Verification items for the finished model (mm, model axes). Round coordinates to 2 decimals unless told otherwise and drop trailing zeros. Order: outer loops, then holes, each group sorted by start corner. A loop starts at its lowest first (then second) coordinate and runs counter-clockwise, first axis right, second up. Notation, with made-up numbers: (66.25, 5.5) -> (80.25, 5.5) arc R20 ccw to (80.25, 22.5) -> close; hole circle Ø7 at (74, 59). An arc over 180 degrees is marked (long way). Return JSON: item names as keys, results as strings. Group by question number.
1) Section check A-A on y = -4. Enter the section's corners in (x, z) (3 decimals), plus the area to 3 significant figures.
2) Depth check by flat-ended pin: pin 1 (1.5 mm diameter, centred on x = -0.5, y = -1.5, fed in from +Z). Enter the tip coordinate at first touch or a pass-through.
3) Scan lines: L1, parallel to Z at x = -0.05, y = -5.25; L2, parallel to Y at x = -0.85, z = 0.65; L3, parallel to Z at x = -0.8, y = -0.25. Record each from-to range of solid material in increasing order.
4) Draft check along X on faces 1 (the cylindrical face through (0.808, -4.169, -0.335)), 2 (the flat face through (0, -0.5, 0)), 3 (the flat face through (-0.65, -1.3, -0.98)). Enter one of: pulls with the +X half, pulls with the -X half, needs draft (parallel to the pull), parting line crosses it, or undercut.
```python
from build123d import *

# Parameters (mm, degrees)
CUT_EXTRUDE1_DEPTH = 0.5
CUT_EXTRUDE1_TAPER = 15


with BuildPart() as part:
    # Sketch1 → Revolve1 (revolve)
    with BuildSketch(Plane.XY):
        with BuildLine():
            Line((0.875, -6.964405423), (0.875, -1.45))
            ThreePointArc((0.875, -1.45), (0.918933983, -1.343933983), (1.025, -1.3))
            Line((1.025, -1.3), (1.5, -1.3))
            ThreePointArc((1.5, -1.3), (1.747487373, -1.197487373), (1.85, -0.95))
            Line((1.85, -0.95), (1.85, -0.75))
            ThreePointArc((1.85, -0.75), (1.630330086, -0.219669914), (1.1, 0))
            Line((1.1, 0), (0, 0))
            Line((0, 0), (0, -9.3))
            ThreePointArc((0, -9.3), (0.084334338, -9.274047247), (0.139485899, -9.205169593))
            Line((0.139485899, -9.205169593), (0.734811985, -7.7))
            ThreePointArc((0.734811985, -7.7), (0.839640421, -7.338822324), (0.875, -6.964405423))
        make_face()
    revolve(axis=Axis((0, 0, 0), (0, -1, 0)))

    # Sketch2 → Cut-Extrude1 (cut)
    with BuildSketch(Plane(origin=(0, 0, 0), x_dir=(1, 0, 0), z_dir=(0, 1, 0))):
        Polygon((-0.271382595, 1), (-0.33, 0.33), (-1, 0.271382595), (-1, -0.271382595), (-0.33, -0.33), (-0.271382595, -1), (0.271382595, -1), (0.33, -0.33), (1, -0.271382595), (1, 0.271382595), (0.33, 0.33), (0.271382595, 1), align=None)
    extrude(amount=-CUT_EXTRUDE1_DEPTH, taper=CUT_EXTRUDE1_TAPER, mode=Mode.SUBTRACT)


solid = part.part
```
Check result:
{
 "1": {"outline": "circle Ø1.75 at (0, 0)", "area": "2.41 mm^2"},
 "2": {"pin 1": "z = 1.85"},
 "3": {"L1": "-0.87 to 0.87", "L2": "-1.3 to 0", "L3": "-1.45 to -0.22, 0.22 to 1.45"},
 "4": {"face 1": "parting line crosses it", "face 2": "undercut", "face 3": "needs draft"}
}
